Part model, mm, in its own coordinate system. A direction names the side the tool comes from. Give positions to 0.01 mm unless a question says otherwise; leave off trailing zeros. Write each loop counter-clockwise with the first axis right and the second up, starting at its lowest first coordinate (ties: lowest second). Pieces come first, ordered by that corner, then holes. Notation, with made-up numbers: M 86,50 L 133,50 A22 ccw 133,60 Z; hole C -6.75,62 d7. An arc over 180 degrees is marked long. Use a Markdown table: item, result.
```python
from build123d import *

# Parameters (mm, degrees)
SKETCH_1_W          = 15
SKETCH_1_H          = 30
EXTRUDE_1_DEPTH     = 20
SKETCH_2_W          = 5.7
SKETCH_2_H          = 17
CUT_EXTRUDE_1_DEPTH = 31
SKETCH_3_W          = 8
SKETCH_3_H          = 30
EXTRUDE_2_DEPTH     = 150
SKETCH_4_R          = 2.375
CUT_EXTRUDE_2_DEPTH = 16
SKETCH_5_W          = 30
SKETCH_5_H          = 17.5
EXTRUDE_3_DEPTH     = 27
CUT_EXTRUDE_3_DEPTH = 10
SKETCH_7_W          = 30
SKETCH_7_H          = 15
EXTRUDE_4_DEPTH     = 5.3
CUT_EXTRUDE_4_REACH = 44
SKETCH_8_W          = 11.25
SKETCH_8_H          = 21.625


with BuildPart() as part:
    # 스케치1 → 보스-돌출1 (new body)
    with BuildSketch(Plane(origin=(0, 0, 0), x_dir=(1, 0, 0), z_dir=(0, 1, 0))):
        Rectangle(SKETCH_1_W, SKETCH_1_H)
    extrude(amount=EXTRUDE_1_DEPTH)

    # 스케치2 → 컷-돌출1 (cut, through all)
    with BuildSketch(Plane.XY.offset(15)):
        with Locations((-0.65, 8.5)):
            Rectangle(SKETCH_2_W, SKETCH_2_H)
    extrude(amount=-CUT_EXTRUDE_1_DEPTH, mode=Mode.SUBTRACT)

    # 스케치3 → 보스-돌출2 (add)
    with BuildSketch(Plane(origin=(0, 20, 0), x_dir=(1, 0, 0), z_dir=(0, 1, 0))):
        with Locations((-3.5, 0)):
            Rectangle(SKETCH_3_W, SKETCH_3_H)
    extrude(amount=EXTRUDE_2_DEPTH)

    # 스케치4 → 컷-돌출2 (cut, through all)
    with BuildSketch(Plane(origin=(7.5, 0, 0), x_dir=(0, 0, -1), z_dir=(1, 0, 0))):
        with Locations((0, 11)):
            Circle(SKETCH_4_R)
    extrude(amount=-CUT_EXTRUDE_2_DEPTH, mode=Mode.SUBTRACT)

    # 스케치5 → 보스-돌출3 (add)
    with BuildSketch(Plane.ZY.offset(7.5)):
        with Locations((0, 161.25)):
            Rectangle(SKETCH_5_W, SKETCH_5_H)
    extrude(amount=EXTRUDE_3_DEPTH)

    # 스케치6 → 컷-돌출3 (cut)
    with BuildSketch(Plane(origin=(0, 170, 0), x_dir=(1, 0, 0), z_dir=(0, 1, 0))):
        with BuildLine():
            Line((-34.5, 15), (-34.5, 9.9))
            Line((-34.5, 9.9), (-28.4, 9.9))
            ThreePointArc((-28.4, 9.9), (-18.5, 0), (-28.4, -9.9))
            Line((-28.4, -9.9), (-34.5, -9.9))
            Line((-34.5, -9.9), (-34.5, -15))
            Line((-34.5, -15), (0.5, -15))
            Line((0.5, -15), (0.5, 15))
            Line((0.5, 15), (-34.5, 15))
        make_face()
    extrude(amount=-CUT_EXTRUDE_3_DEPTH, mode=Mode.SUBTRACT)

    # 스케치7 → 보스-돌출4 (add)
    with BuildSketch(Plane(origin=(7.5, 0, 0), x_dir=(0, 0, -1), z_dir=(1, 0, 0))):
        with Locations((0, -7.5)):
            Rectangle(SKETCH_7_W, SKETCH_7_H)
    extrude(amount=-EXTRUDE_4_DEPTH)

    # 스케치8 → 컷-돌출4 (cut, up to next)
    with BuildSketch(Plane(origin=(7.5, 0, 0), x_dir=(0, 0, -1), z_dir=(1, 0, 0)), mode=Mode.PRIVATE) as cut_extrude_4_sk1:
        with Locations((0, -4.1875)):
            Rectangle(SKETCH_8_W, SKETCH_8_H)
    cut_extrude_4_tool1 = extrude(cut_extrude_4_sk1.sketch, amount=-CUT_EXTRUDE_4_REACH, mode=Mode.PRIVATE) & part.part
    add(cut_extrude_4_tool1.solids().sort_by_distance((7.5, -4.1875, 0))[0], mode=Mode.SUBTRACT)


solid = part.part
```
1. Drill centre lines: L1, parallel to X at y = 12, z = 10; L2, parallel to Y at x = 5.45, z = 0 (3 decimals); L3, parallel to Y at x = -4.35, z = 0 (3 decimals). Where is each one in solid material? Low to high.
Findings below:
| item | result |
|---|---|
| L1 | -7.5 to -3.5, 2.2 to 7.5 |
| L2 | 6.625 to 8.625, 13.375 to 20 |
| L3 | 0 to 8.625, 13.375 to 160 |
2. Drop flat-ended pins along their axis: P1, Ø4, axis at x = -8, z = 2, coming from the +Y side; P2, Ø3, axis at x = -32.5, y = 163.5, coming from the +Z side; P3, Ø1, axis at y = 24.5, z = -4.5, coming from the -X side. Give the stop position or say it passes through.
Findings below:
| item | result |
|---|---|
| P1 | y = 160 |
| P2 | z = 9.9 |
| P3 | x = -7.5 |
3. Cut at C-C, the plane x = -25.5. Give the cut face in (y, z), then the cut area to 3 significant figures.
Findings below:
| item | result |
|---|---|
| outline | M 152.5,-15 L 160,-15 L 160,-9.47 L 170,-9.47 L 170,9.47 L 160,9.47 L 160,15 L 152.5,15 Z |
| area | 414 mm2 |
4. Cut at A-A, the plane y = 11. Give the cut face in (x, z) (3 decimals), then the cut area to 3 significant figures.
Findings below:
| item | result |
|---|---|
| outline | M -7.5,-15 L -3.5,-15 L -3.5,-2.375 L -7.5,-2.375 Z; M -7.5,2.375 L -3.5,2.375 L -3.5,15 L -7.5,15 Z; M 2.2,-15 L 7.5,-15 L 7.5,-2.375 L 2.2,-2.375 Z; M 2.2,2.375 L 7.5,2.375 L 7.5,15 L 2.2,15 Z |
| area | 235 mm2 |
5. Two-plate mould, pull along Y, no slides. Class faces 4 (the cylindrical face through (4.887, 13.355, 0.309)), 5 (the cylindrical face through (-18.502, 165.07, -0.218)), 6 (the flat face through (-6, 0, 0)), 7 (the cylindrical face through (-5.472, 13.355, 0.309)): released by +Y, released by -Y, zero draft, split by the parting line, or undercut.
Findings below:
| item | result |
|---|---|
| face 4 | undercut |
| face 5 | zero draft |
| face 6 | released by -Y |
| face 7 | undercut |
6. Cut at B-B, the plane z = 0. Give the cut face in (x, y) (3 decimals), then the cut area to 3 significant figures.
Findings below:
| item | result |
|---|---|
| outline | M -34.5,152.5 L -7.5,152.5 L -7.5,13.375 L -3.5,13.375 L -3.5,17 L 2.2,17 L 2.2,13.375 L 7.5,13.375 L 7.5,20 L 0.5,20 L 0.5,160 L -18.5,160 L -18.5,170 L -34.5,170 Z; M -7.5,0 L -3.5,0 L -3.5,8.625 L -7.5,8.625 Z; M 2.2,6.625 L 7.5,6.625 L 7.5,8.625 L 2.2,8.625 Z |
| area | 1,610 mm2 |
7. Tool access for faces 1 (the flat face through (5, -4, 5.625)), 2 (the flat face through (-1, 17, 0)), 3 (the flat face through (0.5, 89, 0)): list every direction of +Z, -Z, +X, -X, +Y, -Y with a clear straight run to the whole face (end or side of a thin tool).
Findings below:
| item | result |
|---|---|
| face 1 | +X, -Y |
| face 2 | +Z, -Z, -Y |
| face 3 | +Z, -Z, +X, +Y |
8. Cut at D-D, the plane z = 13. Give the cut face in (x, y).
Findings below:
| item | result |
|---|---|
| outline | M -34.5,152.5 L -7.5,152.5 L -7.5,0 L -3.5,0 L -3.5,17 L 2.2,17 L 2.2,-15 L 7.5,-15 L 7.5,20 L 0.5,20 L 0.5,160 L -34.5,160 Z |
